```python
from build123d import *

# Parameters (mm, degrees)
BASE_FLANGE1_DEPTH = 1
SKETCH6_R          = 27.45
CUT_EXTRUDE1_DEPTH = 10
SKETCH8_R          = 2.05
SKETCH8_R_2        = 1.3
CUT_EXTRUDE3_DEPTH = 10
CIRPATTERN2_COUNT  = 4


# Sheet-metal steps are written as plain solids
with BuildPart() as part:
    # Sketch1 → Base-Flange1 (new body)
    with BuildSketch(Plane(origin=(0, 0, 0), x_dir=(1, 0, 0), z_dir=(0, 1, 0))):
        with BuildLine():
            Line((-46.2, -51.2), (46.2, -51.2))
            ThreePointArc((46.2, -51.2), (49.735533906, -49.735533906), (51.2, -46.2))
            Line((51.2, -46.2), (51.2, 46.2))
            ThreePointArc((51.2, 46.2), (49.735533906, 49.735533906), (46.2, 51.2))
            Line((46.2, 51.2), (-46.2, 51.2))
            ThreePointArc((-46.2, 51.2), (-49.735533906, 49.735533906), (-51.2, 46.2))
            Line((-51.2, 46.2), (-51.2, -46.2))
            ThreePointArc((-51.2, -46.2), (-49.735533906, -49.735533906), (-46.2, -51.2))
        make_face()
    extrude(amount=-BASE_FLANGE1_DEPTH)

    # Sketch6 → Cut-Extrude1 (cut)
    with BuildSketch(Plane(origin=(0, 0, 0), x_dir=(1, 0, 0), z_dir=(0, 1, 0))):
        with Locations(Location((0, 0, 0), (0, 0, 270))):
            Circle(SKETCH6_R)
    extrude(amount=-CUT_EXTRUDE1_DEPTH, mode=Mode.SUBTRACT)

    # Sketch8 → Cut-Extrude3 (cut)
    with BuildSketch(Plane(origin=(0, 0, 0), x_dir=(1, 0, 0), z_dir=(0, 1, 0))):
        with Locations(Location((45.02, 45.02, 0), (0, 0, 270))):
            Circle(SKETCH8_R)
        with Locations(Location((37.45, 37.45, 0), (0, 0, 270))):
            Circle(SKETCH8_R_2)
    cut_extrude3 = extrude(amount=-CUT_EXTRUDE3_DEPTH, mode=Mode.SUBTRACT)

    # CirPattern2: Cut-Extrude3 ×4 about axis
    cirpattern2_axis = Axis((0, 0, 0), (0, 1, 0))
    for i in range(1, CIRPATTERN2_COUNT):
        add(cut_extrude3.rotate(cirpattern2_axis, i * 360 / CIRPATTERN2_COUNT), mode=Mode.SUBTRACT)


solid = part.part
```
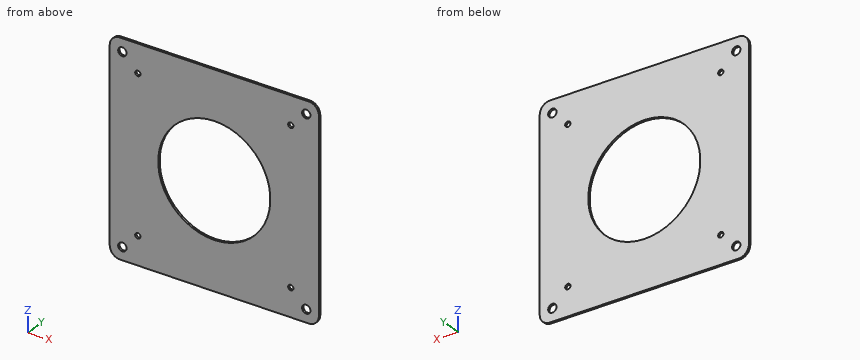
Can you work these out from the model? Positions are in its coordinate system, mm. Give positions to 0.01 mm unless a question says otherwise; leave off trailing zeros. Order: outer loops, then holes, each group sorted by start corner. A loop starts at its lowest first (then second) coordinate and runs counter-clockwise, first axis right, second up. Notation, with made-up numbers: M 40.25,-24.75 L 71.25,-24.75 A35 cw 71.25,14.25 Z; hole C 32.5,79.5 d1. An arc over 180 degrees is marked long. One line per item, written item: value.
1) I want a section at D-D, the plane x = 0. List the corners of the cut face in (y, z) for me, plus the area to 3 significant figures.
Answer sheet:
outline: M -1,-51.2 L 0,-51.2 L 0,-27.45 L -1,-27.45 Z; M -1,27.45 L 0,27.45 L 0,51.2 L -1,51.2 Z
area: 47.5 mm^2
2) For P1, Ø3.5, axis at x = 45.02, z = -45.02, coming from the -Y side; P2, Ø4.5, axis at x = -45.02, z = 45.02, coming from the -Y side, each with a flat end and sliding along its axis, tell me the tip position at first contact or that it passes through.
Answer sheet:
P1: passes through
P2: stops at y = -1
3) I want a section at C-C, the plane z = -45.02. List the corners of the cut face in (x, y) for me, plus the area to 3 significant figures.
Answer sheet:
outline: M -51.2,-1 L -47.07,-1 L -47.07,0 L -51.2,0 Z; M -42.97,-1 L 42.97,-1 L 42.97,0 L -42.97,0 Z; M 47.07,-1 L 51.2,-1 L 51.2,0 L 47.07,0 Z
area: 94.2 mm^2
4) I want a section at B-B, the plane z = 0. List the corners of the cut face in (x, y) for me.
Answer sheet:
outline: M -51.2,-1 L -27.45,-1 L -27.45,0 L -51.2,0 Z; M 27.45,-1 L 51.2,-1 L 51.2,0 L 27.45,0 Z
5) I want a section at A-A, the plane x = -45.02. List the corners of the cut face in (y, z) for me.
Answer sheet:
outline: M -1,-51.2 L 0,-51.2 L 0,-47.07 L -1,-47.07 Z; M -1,-42.97 L 0,-42.97 L 0,42.97 L -1,42.97 Z; M -1,47.07 L 0,47.07 L 0,51.2 L -1,51.2 Z
6) Please list where these lines run through material, in increasing order: line 1 along X through (y, z) = (-0.8, -45.02); line 2 along X through (y, z) = (-0.75, -37.45); line 3 along Z through (x, y) = (-1, -0.3).
Answer sheet:
line 1: x = -51.2 to -47.07, -42.97 to 42.97, 47.07 to 51.2
line 2: x = -51.2 to -38.75, -36.15 to 36.15, 38.75 to 51.2
line 3: z = -51.2 to -27.43, 27.43 to 51.2
